```python
from build123d import *

# Parameters (mm, degrees)
SKETCH2_W           = 7.62
SKETCH2_H           = 8.89
SKETCH2_W_2         = 13.97
SKETCH2_H_2         = 44.45
BOSS_EXTRUDE1_DEPTH = 6.35
SKETCH3_R           = 4.0005
CUT_EXTRUDE1_DEPTH  = 2.794
CUT_EXTRUDE2_DEPTH  = 1.5875


with BuildPart() as part:
    # Sketch2 → Boss-Extrude1 (new body)
    with BuildSketch(Plane.XY):
        with Locations((-17.78, 48.895)):
            Rectangle(SKETCH2_W, SKETCH2_H)
        with Locations((-6.985, 48.895)):
            Rectangle(SKETCH2_W_2, SKETCH2_H)
        with Locations((-6.985, 22.225)):
            Rectangle(SKETCH2_W_2, SKETCH2_H_2)
    extrude(amount=BOSS_EXTRUDE1_DEPTH)

    # Sketch3 → Cut-Extrude1 (cut)
    with BuildSketch(Plane(origin=(0, 0, 0), x_dir=(-1, 0, 0), z_dir=(0, 0, -1))):
        with Locations((6.985, 15.24)):
            Circle(SKETCH3_R)
    extrude(amount=-CUT_EXTRUDE1_DEPTH, mode=Mode.SUBTRACT)

    # Sketch4 → Cut-Extrude2 (cut)
    with BuildSketch(Plane(origin=(0, 0, 0), x_dir=(-1, 0, 0), z_dir=(0, 0, -1))):
        Polygon((6.985, 29.718), (9.017, 29.718), (9.017, 15.24), (9.017, 0.762), (4.953, 0.762), (4.953, 15.24), (4.953, 29.718), align=None)
    extrude(amount=-CUT_EXTRUDE2_DEPTH, mode=Mode.SUBTRACT)


solid = part.part
```
Check sheet for the modelled part. Datum: model origin and axes. Units: mm. A direction names the side the tool comes from. Give positions to 0.01 mm unless a question says otherwise; leave off trailing zeros. Order: outer loops, then holes, each group sorted by start corner. A loop starts at its lowest first (then second) coordinate and runs counter-clockwise, first axis right, second up. Notation, with made-up numbers: M 14.25,20 L 58.25,20 A23 ccw 58.25,28 Z; hole C 15.25,68 d1. An arc over 180 degrees is marked long. Answer in a Markdown table with one row per item.
1) Cross-section at B-B, the plane y = 15.24. Enter the section's corners in (x, z), plus the area to 3 significant figures.
Filled sheet:
| item | result |
|---|---|
| outline | M -13.97,0 L -10.99,0 L -10.99,2.79 L -2.98,2.79 L -2.98,0 L 0,0 L 0,6.35 L -13.97,6.35 Z |
| area | 66.4 mm2 |
2) Gauge pin test, flat ends, axial feed: P1, Ø3, axis at y = 28.5, z = 4.5, coming from the -X side; P2, Ø3, axis at x = -16.5, z = 3, coming from the -Y side. Record the tip position at first contact, or that the pin passes through.
Filled sheet:
| item | result |
|---|---|
| P1 | stops at x = -13.97 |
| P2 | stops at y = 44.45 |
3) Access from +Z, -Z, +X, -X, +Y, -Y to the whole of each face (thin tool, end or side, straight path). Record for faces 1 (the flat face through (-9, 33, 0)), 2 (the flat face through (-4.953, 24, 1)), 3 (the flat face through (-18, 44.45, 3)).
Filled sheet:
| item | result |
|---|---|
| face 1 | -Z, +X, -X, +Y, -Y |
| face 2 | -Z |
| face 3 | +Z, -Z, -X, -Y |
4) Thickness scan on L1, parallel to X at y = 4.5, z = 0.75; L2, parallel to Y at x = -9, z = 2.25; L3, parallel to Y at x = -5, z = 1.25. Record the ranges inside material, lowest first. Write a range as [from, to].
Filled sheet:
| item | result |
|---|---|
| L1 | x = [-13.97, -9.02], [-4.95, 0] |
| L2 | y = [0, 11.78], [18.7, 53.34] |
| L3 | y = [0, 0.76], [29.72, 53.34] |
5) Cross-section at C-C, the plane x = -4.25. Enter the section's corners in (y, z), plus the area to 3 significant figures.
Filled sheet:
| item | result |
|---|---|
| outline | M 0,0 L 12.32,0 L 12.32,2.79 L 18.16,2.79 L 18.16,0 L 53.34,0 L 53.34,6.35 L 0,6.35 Z |
| area | 322 mm2 |
6) Cross-section at D-D, the plane z = 5.75. Enter the section's corners in (x, y).
Filled sheet:
| item | result |
|---|---|
| outline | M -21.59,44.45 L -13.97,44.45 L -13.97,0 L 0,0 L 0,53.34 L -21.59,53.34 Z |
